Geometry check sheet. Reference: the model listing, model coordinates, mm. A direction names the side the tool comes from. Coordinates: 2 decimals unless noted, no trailing zeros. Loops run counter-clockwise (first coordinate to the right, second up) from the corner with the lowest first, then second, coordinate; pieces in that order, holes last. Notation, with made-up numbers: (18.25, 57.25) - (58.25, 57.25) arc R28 ccw to (58.25, 82.25) - close; hole circle Ø3 at (-30, -3.5). An arc over 180 degrees is marked (long way). Write each question's results on one line, items separated by ' | '. Start each with the question number.
(1) Sectioned sample at A-A (x = 0). Enter the section's corners in (y, z), plus the area to 3 significant figures.
(2) Sectioned sample at D-D (x = -16.5). Enter the section's corners in (y, z), plus the area to 3 significant figures.
(3) Material ranges on probe 1 along Y at (x, z) = (0, 1.05); probe 2 along X at (y, z) = (-1.5, 0.6); probe 3 along Z at (x, y) = (14, -0.25), recorded low to high.
(4) Sectioned sample at B-B (y = 0). Enter the section's corners in (x, z).
(5) Access from +Z, -Z, +X, -X, +Y, -Y to the whole of each face (thin tool, end or side, straight path). Record for faces 1 (the face through (-0.867, -3.905, 3.479)), 2 (the face through (0, 6, 1)).
(6) Sectioned sample at C-C (z = 3.7). Enter the section's corners in (x, y).
(7) Mould release check, pull along X, two halves, no side actions. Record for faces 3 (the face through (4.5, 0.1, 2)), 4 (the face through (19, -0.5, 1)), 5 (the face through (-9.15, 4.37, 0.99)), 6 (the face through (-1, 1, 2)): pulls with the +X half, pulls with the -X half, needs draft (parallel to the pull), parting line crosses it, or undercut.
(8) Go/stop test with flat-tipped pins: pin 1 Ø1 at (x, z) = (-5.5, 1.5) entering from -Y; pin 2 Ø4.5 at (x, y) = (0, 0) entering from +Z. Record where each tip stops, or that it passes through.
from build123d import *

# Parameters (mm, degrees)
SKETCH1_R           = 1.25
BOSS_EXTRUDE1_DEPTH = 2
SKETCH2_R           = 4
SKETCH2_R_2         = 2.5
BOSS_EXTRUDE2_DEPTH = 3


with BuildPart() as part:
    # Sketch1 → Boss-Extrude1 (new body)
    with BuildSketch(Plane.XY):
        with BuildLine():
            Line((-16.965907586, 2.88879085), (-1.118178206, 5.894885707))
            ThreePointArc((-1.118178206, 5.894885707), (0.157250865, 5.997938993), (1.425527907, 5.828196135))
            Line((1.425527907, 5.828196135), (17.093969961, 1.995826584))
            ThreePointArc((17.093969961, 1.995826584), (18.999141247, -0.498109666), (16.965907586, -2.88879085))
            Line((16.965907586, -2.88879085), (1.118178206, -5.894885707))
            ThreePointArc((1.118178206, -5.894885707), (-0.157250865, -5.997938993), (-1.425527907, -5.828196135))
            Line((-1.425527907, -5.828196135), (-17.093969961, -1.995826584))
            ThreePointArc((-17.093969961, -1.995826584), (-18.999141247, 0.498109666), (-16.965907586, 2.88879085))
        make_face()
        with Locations((-16.5, 0.432588472)):
            Circle(SKETCH1_R, mode=Mode.SUBTRACT)
        with Locations((16.5, -0.432588472)):
            Circle(SKETCH1_R, mode=Mode.SUBTRACT)
        Circle(SKETCH1_R, mode=Mode.SUBTRACT)
    extrude(amount=BOSS_EXTRUDE1_DEPTH)

    # Sketch2 → Boss-Extrude2 (add)
    with BuildSketch(Plane.XY.offset(2)):
        Circle(SKETCH2_R)
        Circle(SKETCH2_R_2, mode=Mode.SUBTRACT)
    extrude(amount=BOSS_EXTRUDE2_DEPTH)


solid = part.part
Outcome:
1) outline: (-6, 0) - (-1.25, 0) - (-1.25, 2) - (-2.5, 2) - (-2.5, 5) - (-4, 5) - (-4, 2) - (-6, 2) - close; (1.25, 0) - (6, 0) - (6, 2) - (4, 2) - (4, 5) - (2.5, 5) - (2.5, 2) - (1.25, 2) - close | area: 28.0 mm2
2) outline: (-2.14, 0) - (-0.82, 0) - (-0.82, 2) - (-2.14, 2) - close; (1.68, 0) - (2.98, 0) - (2.98, 2) - (1.68, 2) - close | area: 5.24 mm2
3) probe 1: y = -6 to -1.25, 1.25 to 6 | probe 2: x = -18.09 to 15.85, 17.15 to 18.76 | probe 3: z = 0 to 2
4) outline: (-18.96, 0) - (-17.67, 0) - (-17.67, 2) - (-18.96, 2) - close; (-15.33, 0) - (-1.25, 0) - (-1.25, 2) - (-2.5, 2) - (-2.5, 5) - (-4, 5) - (-4, 2) - (-15.33, 2) - close; (1.25, 0) - (15.33, 0) - (15.33, 2) - (4, 2) - (4, 5) - (2.5, 5) - (2.5, 2) - (1.25, 2) - close; (17.67, 0) - (18.96, 0) - (18.96, 2) - (17.67, 2) - close
5) face 1: +Z | face 2: +Z, -Z, +Y
6) outline: circle Ø8 at (0, 0); hole circle Ø5 at (0, 0)
7) face 3: needs draft | face 4: pulls with the +X half | face 5: pulls with the -X half | face 6: undercut
8) pin 1: stops at y = -4.95 | pin 2: stops at z = 2
